```python
from build123d import *

# Parameters (mm, degrees)
ESQUISSE1_W        = 11.8
ESQUISSE1_H        = 22.5
BOSS_EXTRU_1_DEPTH = 15.9
BOSS_EXTRU_2_DEPTH = 2.5
ESQUISSE4_W        = 11.8
ESQUISSE4_H        = 22.5
BOSS_EXTRU_3_DEPTH = 4.3
BOSS_EXTRU_4_DEPTH = 4
ESQUISSE6_R        = 2.3
ESQUISSE6_R_2      = 0.85
BOSS_EXTRU_5_DEPTH = 3.2
CONG_1_R           = 0.2


with BuildPart() as part:
    # Esquisse1 → Boss.-Extru.1 (new body)
    with BuildSketch(Plane(origin=(0, 0, 0), x_dir=(1, 0, 0), z_dir=(0, 1, 0))):
        Rectangle(ESQUISSE1_W, ESQUISSE1_H)
    extrude(amount=BOSS_EXTRU_1_DEPTH)

    # Esquisse3 → Boss.-Extru.2 (add)
    with BuildSketch(Plane(origin=(0, 15.9, 0), x_dir=(1, 0, 0), z_dir=(0, 1, 0))):
        with BuildLine():
            Line((-5.9, 15.95), (-5.9, -15.95))
            Line((-5.9, -15.95), (-0.65, -15.95))
            Line((-0.65, -15.95), (-0.65, -14.409934208))
            ThreePointArc((-0.65, -14.409934208), (0, -12.65), (0.65, -14.409934208))
            Line((0.65, -14.409934208), (0.65, -15.95))
            Line((0.65, -15.95), (5.9, -15.95))
            Line((5.9, -15.95), (5.9, 15.95))
            Line((5.9, 15.95), (0.65, 15.95))
            Line((0.65, 15.95), (0.65, 14.409934208))
            ThreePointArc((0.65, 14.409934208), (0, 12.65), (-0.65, 14.409934208))
            Line((-0.65, 14.409934208), (-0.65, 15.95))
            Line((-0.65, 15.95), (-5.9, 15.95))
        make_face()
    extrude(amount=BOSS_EXTRU_2_DEPTH)

    # Esquisse4 → Boss.-Extru.3 (add)
    with BuildSketch(Plane(origin=(0, 18.4, 0), x_dir=(1, 0, 0), z_dir=(0, 1, 0))):
        Rectangle(ESQUISSE4_W, ESQUISSE4_H)
    extrude(amount=BOSS_EXTRU_3_DEPTH)

    # Esquisse5 → Boss.-Extru.4 (add)
    with BuildSketch(Plane(origin=(0, 22.7, 0), x_dir=(1, 0, 0), z_dir=(0, 1, 0))):
        with BuildLine():
            Line((2.5, -0.95), (2.5, 0.005844314))
            ThreePointArc((2.5, 0.005844314), (0, 11.25), (-2.5, 0.005844314))
            Line((-2.5, 0.005844314), (-2.5, -0.95))
            ThreePointArc((-2.5, -0.95), (0, -3.45), (2.5, -0.95))
        make_face()
    extrude(amount=BOSS_EXTRU_4_DEPTH)

    # Esquisse6 → Boss.-Extru.5 (add)
    with BuildSketch(Plane(origin=(0, 26.7, 0), x_dir=(1, 0, 0), z_dir=(0, 1, 0))):
        with Locations((0, 5.35)):
            Circle(ESQUISSE6_R)
        with Locations((0, 5.35)):
            Circle(ESQUISSE6_R_2, mode=Mode.SUBTRACT)
    extrude(amount=BOSS_EXTRU_5_DEPTH)

    # Congé1
    cong_1_edges = [part.edges().sort_by_distance(p)[0] for p in [
        (0, 0, -11.25),
        (-5.9, 17.15, -15.95),
        (5.9, 17.15, -15.95),
        (5.9, 15.9, -13.6),
        (5.9, 18.4, -13.6),
        (5.9, 20.55, -11.25),
        (-5.9, 20.55, -11.25),
        (3.275, 18.4, -15.95),
        (3.275, 15.9, -15.95),
        (-3.275, 18.4, -15.95),
        (-3.275, 15.9, -15.95),
        (-5.9, 15.9, -13.6),
        (-5.9, 18.4, -13.6),
        (5.9, 20.55, 11.25),
        (0, 22.7, 11.25),
        (-5.9, 20.55, 11.25),
        (5.9, 18.4, 13.6),
        (5.9, 15.9, 13.6),
        (5.9, 17.15, 15.95),
        (3.275, 18.4, 15.95),
        (3.275, 15.9, 15.95),
        (-5.9, 17.15, 15.95),
        (-3.275, 18.4, 15.95),
        (-3.275, 15.9, 15.95),
        (-5.9, 15.9, 13.6),
        (-5.9, 18.4, 13.6),
        (5.9, 7.95, -11.25),
        (5.9, 0, 0),
        (5.9, 7.95, 11.25),
        (0, 0, 11.25),
        (-5.9, 7.95, 11.25),
        (-5.9, 0, 0),
        (-5.9, 7.95, -11.25),
    ]]
    fillet(cong_1_edges, radius=CONG_1_R)


solid = part.part
```
Here's how the part is built. I have some questions about the finished solid (model axes, mm). A direction names the side the tool comes from. Coordinates: 2 decimals unless noted, no trailing zeros. Write each loop counter-clockwise with the first axis right and the second up, starting at its lowest first coordinate (ties: lowest second). Pieces come first, ordered by that corner, then holes. Notation, with made-up numbers: (-0.75, 80) -> (14.25, 80) arc R13 ccw to (14.25, 95) -> close; hole circle Ø9 at (-16, 28.25). An arc over 180 degrees is marked (long way). Use a Markdown table: item, result. Add a question column.
(1) For faces 1 (the flat face through (0, 8, -11.25)), 2 (the flat face through (-0.1, 18.4, -12.5)), 3 (the flat face through (4, 22.7, -10)), which set-ups out of +Z, -Z, +X, -X, +Y, -Y let a thin tool reach every point of the face, with its end or its side?
(2) If we section it at A-A, the plane z = -13.65: Write out the boundary of the cut face in (x, y).
(3) If we section it at B-B, the plane y = 3: Write out the boundary of the cut face in (x, z).
(4) If we section it at C-C, the plane z = 9: Write out the boundary of the cut face in (x, y), and give its area (3 significant figures).
(5) I'm going to push flat-ended pins straight in: P1, Ø3.5, axis at x = 0, y = 9, coming from the -Z side; P2, Ø3.5, axis at x = -0.5, z = 12.5, coming from the +Y side; P3, Ø1, axis at x = -3, z = -10, coming from the +Y side. Where does each tip first touch, or does it pass through?
(6) Please list where these lines run through material, in increasing order: line 1 (X direction, y = 27.55, z = -5.35); line 2 (X direction, y = 16.7, z = -13.65); line 3 (Z direction, x = 0, y = 28.2).
(7) We'd pull the mould along Z, two halves only. Please class faces 4 (the flat face through (-3, 17, 15.95)), 5 (the flat face through (0, 26.7, -5)), 6 (the flat face through (-2.5, 24.7, 0.5)): +Z half, -Z half, draft (parallel to the pull), parting line (faces both ways), or undercut.
(8) If we section it at D-D, the plane x = 4.25: Write out the boundary of the cut face in (y, z), and give its area (3 significant figures).
Outcome:
| question | item | result |
|---|---|---|
| 1 | face 1 | -Z, +X, -X, -Y |
| 1 | face 2 | -Z, +X, -X, +Y |
| 1 | face 3 | -Z, +X, +Y |
| 2 | outline | (-5.9, 16.1) arc R0.2 ccw to (-5.7, 15.9) -> (-1, 15.9) -> (-1, 18.4) -> (-5.7, 18.4) arc R0.2 ccw to (-5.9, 18.2) -> close; (1, 15.9) -> (5.7, 15.9) arc R0.2 ccw to (5.9, 16.1) -> (5.9, 18.2) arc R0.2 ccw to (5.7, 18.4) -> (1, 18.4) -> close |
| 3 | outline | (-5.9, -11.05) arc R0.2 ccw to (-5.7, -11.25) -> (5.7, -11.25) arc R0.2 ccw to (5.9, -11.05) -> (5.9, 11.05) arc R0.2 ccw to (5.7, 11.25) -> (-5.7, 11.25) arc R0.2 ccw to (-5.9, 11.05) -> close |
| 4 | outline | (-5.9, 0.2) arc R0.2 ccw to (-5.7, 0) -> (5.7, 0) arc R0.2 ccw to (5.9, 0.2) -> (5.9, 22.7) -> (-5.9, 22.7) -> close |
| 4 | area | 268 mm^2 |
| 5 | P1 | stops at z = -11.25 |
| 5 | P2 | stops at y = 22.7 |
| 5 | P3 | stops at y = 26.7 |
| 6 | line 1 | x = -2.3 to -0.85, 0.85 to 2.3 |
| 6 | line 2 | x = -5.9 to -1, 1 to 5.9 |
| 6 | line 3 | z = -7.65 to -6.2, -4.5 to -3.05 |
| 7 | face 4 | +Z half |
| 7 | face 5 | undercut |
| 7 | face 6 | draft |
| 8 | outline | (0, -11.05) arc R0.2 ccw to (0.2, -11.25) -> (15.9, -11.25) -> (15.9, -15.75) arc R0.2 ccw to (16.1, -15.95) -> (18.2, -15.95) arc R0.2 ccw to (18.4, -15.75) -> (18.4, -11.25) -> (22.7, -11.25) -> (22.7, -9.44) -> (26.7, -9.44) -> (26.7, -1.26) -> (22.7, -1.26) -> (22.7, 11.05) arc R0.2 ccw to (22.5, 11.25) -> (18.4, 11.25) -> (18.4, 15.75) arc R0.2 ccw to (18.2, 15.95) -> (16.1, 15.95) arc R0.2 ccw to (15.9, 15.75) -> (15.9, 11.25) -> (0.2, 11.25) arc R0.2 ccw to (0, 11.05) -> close |
| 8 | area | 567 mm^2 |
